Can you work these out from the model? Positions are in its coordinate system, mm. Face numbers are marked on the shaded views. A direction names the side the tool comes from. Coordinates: 2 decimals unless noted, no trailing zeros. Order: outer loops, then holes, each group sorted by start corner. A loop starts at its lowest first (then second) coordinate and runs counter-clockwise, first axis right, second up. Notation, with made-up numbers: (58.5, -38) -> (71.5, -38) arc R18 ccw to (71.5, -5) -> close; hole circle Ø11 at (88.5, 80). An arc over 180 degrees is marked (long way). Answer in a Markdown table with one row per item. Add a question column.
1. Imagine slicing it at C-C on y = 3.75. Write out the boundary of the cut face in (x, z), plus the area to 3 significant figures.
2. Imagine slicing it at A-A on x = -15. Write out the boundary of the cut face in (y, z), plus the area to 3 significant figures.
3. On a 3-axis mill with a long thin cutter (end or side, diameter ignored), from which of +Z, -Z, +X, -X, +Y, -Y can I reach the whole of each face in a straight line? I mean the marked faces 4 and 5. Say none if no direction works.
4. If I drill on line 1 along X through (y, z) = (2.5, 0); line 2 along Z through (x, y) = (-6.5, 6.75); line 3 along Z through (x, y) = (-7.5, 3), over which ranges is the centre line in solid material (lowest first)? Write a range as [from, to].
5. Imagine slicing it at B-B on z = 0. Write out the boundary of the cut face in (x, y), plus the area to 3 significant figures.
6. We'd pull the mould along Z, two halves only. Please class the marked faces 1, 2 and 3: pulls with the +Z half, pulls with the -Z half, needs draft (parallel to the pull), parting line crosses it, or undercut.
7. Will these pins go through, and if not, where does the flat tip stop? pin 1 (8 mm diameter, centred on x = -7.5, z = 15, fed in from -Y); pin 2 (1 mm diameter, centred on x = 15.5, y = 8, fed in from -Z); pin 3 (5 mm diameter, centred on x = 17, y = 7, fed in from +Z); pin 4 (2.5 mm diameter, centred on x = -1.5, y = 5, fed in from -Z).
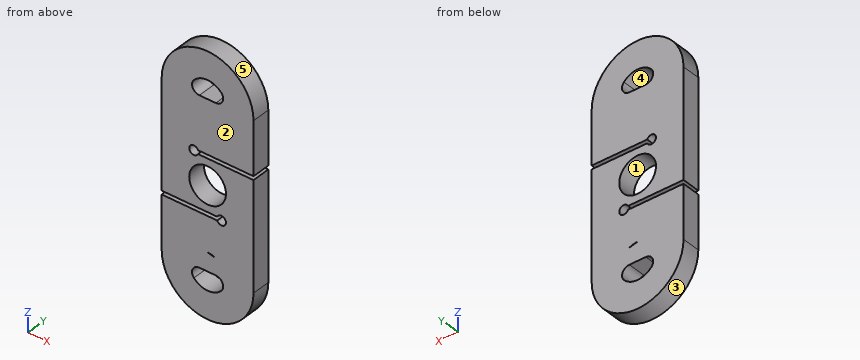
Autodesk Inventor part; units mm, degrees
ref_plane "YZ Plane" through (0, 0, 0) normal (1, 0, 0) x (0, 1, 0)
ref_plane "XZ Plane" through (0, 0, 0) normal (0, 1, 0) x (-1, 0, 0)
ref_plane "XY Plane" through (0, 0, 0) normal (0, 0, 1) x (1, 0, 0)
sketch "Boceto1" plane through (0, 0, 0) normal (0, 1, 0) x (-1, 0, 0)
  circle A0 centre (0, -45) radius 10
  circle A1 centre (0, 45) radius 10
  line L0 (0.0371, -35.0001) -> (-0.0371, -35.0001)
  line L1 (0.0371, -35.0001) -> (-4.4959, -36.0676)
  circle A2 centre (0, -45) radius 25
  circle A3 centre (0, 45) radius 25
  line L2 (0, 89.4288) -> (0, -73.1924) construction
  line L3 (-38.8142, 0) -> (36.7218, 0) construction
  line L4 (0, 45) -> (0, -45)
  line L5 (10, 45) -> (-10, 45)
  line L6 (10, -45) -> (-10, -45)
  line L7 (25, 45) -> (25, -45)
  line L8 (-25, -45) -> (-25, 45)
  circle A4 centre (0, 0) radius 10
  circle A5 centre (7.5, 15) radius 2.5
  line L9 (-25, 14) -> (5.2087, 14)
  line L10 (5.2087, 14) -> (5.2087, 16)
  line L11 (5.2087, 16) -> (-25, 16)
  line L12 (-25, 16) -> (-25, 14)
  line L13 (-25, 14) -> (5.2087, 16) construction
  line L14 (5.2087, 14) -> (-25, 16) construction
  line L15 (10, 0) -> (10, 38.9395) construction
  circle A6 centre (-7.5, -15) radius 2.5
  line L16 (25, -16) -> (-5.2087, -16)
  line L17 (-5.2087, -16) -> (-5.2087, -14)
  line L18 (-5.2087, -14) -> (25, -14)
  line L19 (25, -14) -> (25, -16)
  line L20 (25, -16) -> (-5.2087, -14) construction
  line L21 (-5.2087, -16) -> (25, -14) construction
  line L22 (-10, 0) -> (-10, -29.6504) construction
  point P0 (0, 60)
  point P1 (0, -60)
  point P2 (-0.0332, 54.9999)
  point P3 (-0.0332, 54.9999)
  point P4 (-12.4808, 36.6795)
  point P5 (11.1803, 35)
  point P6 (-9.8956, 15)
  point P7 (-9.8956, 15)
  point P8 (-25, 15)
  point P9 (9.8956, -15)
  point P10 (9.8956, -15)
  point P11 (25, -15)
  point P12 (25, -16)
  point P13 (-5.2087, -16)
  point P14 (25, -14)
  point P15 (5.2087, 14)
  dimension "d48" = 5
  dimension "d51" = 5
  dimension "d42" = 50
  dimension "d43" = 50
  dimension "d44" = 90
  dimension "d45" = 20
  dimension "d46" = 20
  dimension "d47" = 20
  dimension "d49" = 2
  dimension "d50" = 14
  dimension "d52" = 2
  dimension "d53" = 14
extrude "Extrusión9" add sketch "Boceto1" along normal blind 10 contours L6 L4 L1 A0 | A2 | A2 L8 L9 L4 A4 L18 A6 L16 | L4 L16 L7 A2 | A0 L1 L4 L6 | L4 A4 L9 A5 L11 A3 L7 L18 | L8 A3 L4 L11 | A1 L5 L4 | L4 L5 A1 | A3
fillet "Empalme3" radius 4 4 edges at (-10, 5, -45) (10, 5, -45) (-10, 5, 45) (10, 5, 45)
properties part number "mod6" material "Aluminio 6061"
Answers follow:
| question | item | result |
|---|---|---|
| 1 | outline | (-25, -45) arc R25 ccw to (25, -45) -> (25, 14) -> (-5.21, 14) arc R2.5 cw (long way) to (-5.21, 16) -> (25, 16) -> (25, 45) arc R25 ccw to (-25, 45) -> (-25, -14) -> (5.21, -14) arc R2.5 cw (long way) to (5.21, -16) -> (-25, -16) -> close; hole circle Ø20 at (0, 0); hole (-7.45, -51.67) arc R10 ccw to (7.45, -51.67) arc R4 ccw to (4.47, -45) -> (-4.47, -45) arc R4 ccw to start; hole (-7.45, 51.67) arc R4 ccw to (-4.47, 45) -> (4.47, 45) arc R4 ccw to (7.45, 51.67) arc R10 ccw to start; hole (-0.04, -35) -> (4.5, -36.07) arc R10 ccw to start |
| 1 | area | 5,710 mm² |
| 2 | outline | (0, -65) -> (10, -65) -> (10, -16) -> (0, -16) -> close; (0, -14) -> (10, -14) -> (10, 65) -> (0, 65) -> close |
| 2 | area | 1,280 mm² |
| 3 | face 4 | +Y, -Y |
| 3 | face 5 | +Z, +Y, -Y |
| 4 | line 1 | x = [-25, -10], [10, 25] |
| 4 | line 2 | z = [-69.14, -52.6], [-45.55, -16], [-14, -7.6], [7.6, 12.71], [17.29, 45.55], [52.6, 69.14] |
| 4 | line 3 | z = [-68.85, -51.61], [-46.39, -16], [-14, -6.61], [6.61, 12.5], [17.5, 46.39], [51.61, 68.85] |
| 5 | outline | (-25, 0) -> (-10, 0) -> (-10, 10) -> (-25, 10) -> close; (10, 0) -> (25, 0) -> (25, 10) -> (10, 10) -> close |
| 5 | area | 300 mm² |
| 6 | face 1 | undercut |
| 6 | face 2 | needs draft |
| 6 | face 3 | pulls with the -Z half |
| 7 | pin 1 | stops at y = 0 |
| 7 | pin 2 | stops at z = -65 |
| 7 | pin 3 | stops at z = 65.37 |
| 7 | pin 4 | stops at z = -70 |
